```python
from build123d import *

# Parameters (mm, degrees)
F0_W     = 68.205244
F0_H     = 92.397712
F1_DEPTH = 25.4
F2_R     = 12.682951
F3_DEPTH = 25.401
F4_W     = 69.079674
F4_H     = 20.986233
F5_DEPTH = 50.8
F6_W     = 17.488527
F6_H     = 13.407867
F7_DEPTH = 46.49133


with BuildPart() as f1:
    # F0 (on Front) → F1 (new body)
    with BuildSketch(Plane.XZ):
        with BuildLine():
            ThreePointArc((0, 75.929344), (-23.81299, 68.820144), (-34.102622, 46.198856))
            Line((-34.102622, 46.198856), (34.102622, 46.198856))
            ThreePointArc((34.102622, 46.198856), (23.81299, 68.820144), (0, 75.929344))
        make_face()
        Rectangle(F0_W, F0_H)
    extrude(amount=F1_DEPTH)

    # F2 (on Front) → F3 (cut, through all)
    with BuildSketch(Plane.XZ):
        with Locations((0, 54.785658)):
            Circle(F2_R)
    extrude(amount=F3_DEPTH, mode=Mode.SUBTRACT)

    # F4 (on Front) → F5 (join)
    with BuildSketch(Plane.XZ):
        with Locations((-0.145737, -35.997214)):
            Rectangle(F4_W, F4_H)
    extrude(amount=F5_DEPTH)

    # F6 (on Top) → F7 (cut, through all)
    with BuildSketch(Plane.XY):
        with Locations((30.896394, -47.073276)):
            Rectangle(F6_W, F6_H)
    extrude(amount=-F7_DEPTH, mode=Mode.SUBTRACT)


solid = f1.part
```
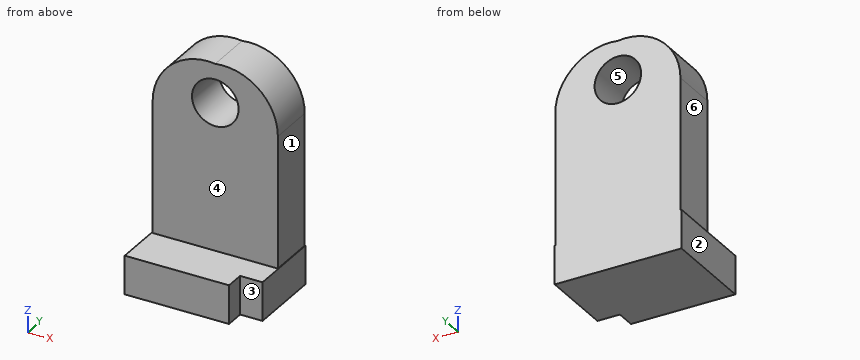
Model file for the job. Use its own axes, mm. Face numbers are marked on the shaded views. A direction names the side the tool comes from. Coordinates: 2 decimals unless noted, no trailing zeros. Write each loop counter-clockwise with the first axis right and the second up, starting at its lowest first coordinate (ties: lowest second). Pieces come first, ordered by that corner, then holes. Notation, with made-up numbers: (49, 35) - (104, 35) arc R7 ccw to (104, 47) - close; hole circle Ø3 at (83.5, 46.25). An arc over 180 degrees is marked (long way). One line per item, written item: value. Start each with the question number.
1. Slice it at C-C (z = -27). Write the cut outline in (x, y).
2. Tool access for the marked faces 1, 2 and 3: list every direction of +Z, -Z, +X, -X, +Y, -Y with a clear straight run to the whole face (end or side of a thin tool).
3. Slice it at D-D (y = -42). Write the cut outline in (x, z).
4. Mould opens along X. For the marked faces 4, 5 and 6 say: released by +X, released by -X, zero draft, split by the parting line, or undercut.
5. Probe line 1 (X direction, y = -46, z = -40.5); line 2 (Y direction, x = -16.5, z = 41); line 3 (X direction, y = -18, z = 44.5). List the from-to ranges inside material, lowest first. Write a range as from..to.
6. Slice it at A-A (x = 9.5). Write the cut outline in (y, z), plus the area to 3 significant figures.
7. Flat gauge pins, fed straight in: pin 1 (3 mm diameter, centred on x = -4, y = -38.5, fed in from +Z); pin 2 (20.5 mm diameter, centred on x = 8, z = 24.5, fed in from -Y); pin 3 (3.5 mm diameter, centred on x = 30.5, z = -34, fed in from -Y). Where does each tip first touch, or does it go through?
8. Slice it at B-B (y = -15). Write the cut outline in (x, z), plus the area to 3 significant figures.
Answers below:
1. outline: (-34.69, -50.8) - (22.15, -50.8) - (22.15, -40.37) - (34.39, -40.37) - (34.39, 0) - (-34.69, 0) - close
2. face 1: +Z, +X, +Y, -Y
2. face 2: +Z, -Z, -X, +Y, -Y
2. face 3: +Z, -Z, +X, -Y
3. outline: (-34.69, -46.49) - (22.15, -46.49) - (22.15, -25.5) - (-34.69, -25.5) - close
4. face 4: zero draft
4. face 5: undercut
4. face 6: released by -X
5. line 1: x = -34.69..22.15
5. line 2: y = -25.4..0
5. line 3: x = -34.1..-7.42, 7.42..34.1
6. outline: (-50.8, -46.49) - (0, -46.49) - (0, 46.38) - (-25.4, 46.38) - (-25.4, -25.5) - (-50.8, -25.5) - close; (-25.4, 63.19) - (0, 63.19) - (0, 75.72) - (-25.4, 75.72) - close
6. area: 3,210 mm^2
7. pin 1: stops at z = -25.5
7. pin 2: stops at y = -25.4
7. pin 3: stops at y = -40.37
8. outline: (-34.69, -46.49) - (34.39, -46.49) - (34.39, -25.5) - (34.1, -25.5) - (34.1, 46.2) arc R30.01 ccw to (0, 75.93) arc R30.01 ccw to (-34.1, 46.2) - (-34.1, -25.5) - (-34.69, -25.5) - close; hole circle Ø25.37 at (0, 54.79)
8. area: 7,490 mm^2
